```python
from build123d import *

# Parameters (mm, degrees)
CYLINDER004_R     = 1.8
CYLINDER004_DEPTH = 10
CYLINDER005_R     = 1.8
CYLINDER005_DEPTH = 10
CYLINDER002_R     = 1.8
CYLINDER002_DEPTH = 10
CYLINDER003_R     = 1.8
CYLINDER003_DEPTH = 10
CYLINDER001_R     = 2.5
CYLINDER001_DEPTH = 24
CYLINDER_R        = 11
CYLINDER_DEPTH    = 2
BOX_W             = 42.3
BOX_H             = 39.8
BOX_DEPTH         = 42.3


with BuildPart() as cylinder004:
    # Cylinder004 → Cylinder004 (new body)
    with BuildSketch(Plane(origin=(5.65, 0, 36.65), x_dir=(1, 0, 0), z_dir=(0, -1, 0))):
        Circle(CYLINDER004_R)
    extrude(amount=CYLINDER004_DEPTH)


with BuildPart() as cylinder005:
    # Cylinder005 → Cylinder005 (new body)
    with BuildSketch(Plane(origin=(36.65, 0, 36.65), x_dir=(1, 0, 0), z_dir=(0, -1, 0))):
        Circle(CYLINDER005_R)
    extrude(amount=CYLINDER005_DEPTH)


with BuildPart() as cylinder002:
    # Cylinder002 → Cylinder002 (new body)
    with BuildSketch(Plane(origin=(5.65, 0, 5.65), x_dir=(1, 0, 0), z_dir=(0, -1, 0))):
        Circle(CYLINDER002_R)
    extrude(amount=CYLINDER002_DEPTH)


with BuildPart() as cylinder003:
    # Cylinder003 → Cylinder003 (new body)
    with BuildSketch(Plane(origin=(36.65, 0, 5.65), x_dir=(1, 0, 0), z_dir=(0, -1, 0))):
        Circle(CYLINDER003_R)
    extrude(amount=CYLINDER003_DEPTH)


with BuildPart() as cylinder001:
    # Cylinder001 → Cylinder001 (new body)
    with BuildSketch(Plane(origin=(21.15, -2, 21.15), x_dir=(1, 0, 0), z_dir=(0, -1, 0))):
        Circle(CYLINDER001_R)
    extrude(amount=CYLINDER001_DEPTH)


with BuildPart() as cylinder:
    # Cylinder → Cylinder (new body)
    with BuildSketch(Plane(origin=(21.15, 0, 21.15), x_dir=(1, 0, 0), z_dir=(0, -1, 0))):
        Circle(CYLINDER_R)
    extrude(amount=CYLINDER_DEPTH)


with BuildPart() as fusion002:
    # Box → Box (new body)
    with BuildSketch(Plane.XY):
        with Locations((21.15, 19.9)):
            Rectangle(BOX_W, BOX_H)
    extrude(amount=BOX_DEPTH)

    # Fusion: union Cylinder
    add(cylinder.part)

    # Fusion001: union Cylinder001
    add(cylinder001.part)

    # Fusion002: union Cylinder004, Cylinder005, Cylinder002, Cylinder003
    add(cylinder004.part)
    add(cylinder005.part)
    add(cylinder002.part)
    add(cylinder003.part)


solid = fusion002.part
```
Input: part model. Units: mm. Frame: model coordinates. A direction names the side the tool comes from. Give positions to 0.01 mm unless a question says otherwise; leave off trailing zeros. Write each loop counter-clockwise with the first axis right and the second up, starting at its lowest first coordinate (ties: lowest second). Pieces come first, ordered by that corner, then holes. Notation, with made-up numbers: (-30.75, 61) - (-17.75, 61) arc R13 cw to (-17.75, 74) - close; hole circle Ø3 at (88, -18). An arc over 180 degrees is marked (long way). Write item = value, one per line. Start each with the question number.
1. Access query for faces 1 (the flat face through (30, 0, 30)), 2 (the flat face through (0, 20, 21)). Directions: +Z, -Z, +X, -X, +Y, -Y. A direction counts if a zero-diameter tool reaches every point of the face in a straight line with its end or side. Return the directions, or none.
2. First-contact query: pin 1 Ø3 at (x, z) = (36.5, 36.5) entering from -Y; pin 2 Ø1 at (x, z) = (14, 9) entering from -Y; pin 3 Ø3 at (y, z) = (-10.5, 34) entering from +X. Flat tips, straight axial feed; report the tip coordinate or a pass-through.
3. Section query D-D, the plane y = -13. Output: boundary loops of the cut face in (x, z), then the cut area to 3 significant figures.
4. Section query B-B, the plane z = 5.65. Output: boundary loops of the cut face in (x, y).
5. Section query A-A, the plane y = -6. Output: boundary loops of the cut face in (x, z).
6. Ray query, L1, parallel to Y at x = 6, z = 21.5; L2, parallel to Z at x = 7, y = -7; L3, parallel to X at y = -4.5, z = 4. Return the intervals inside material, ascending.
7. Mould query, pull axis X, two halves, no side actions, for faces 3 (the flat face through (6, -10, 37)), 4 (the cylindrical face through (13.04, -0.99, 28.58)), 5 (the cylindrical face through (38.313, -4.93, 35.961)), 6 (the cylindrical face through (38.367, -4.93, 6.191)). Classes: released by +X, released by -X, zero draft, split by the parting line, or undercut.
8. Section query C-C, the plane x = 5.65. Output: boundary loops of the cut face in (y, z), then the cut area to 3 significant figures.
Check sheet entries:
q1.face_1 = -Y
q1.face_2 = +Z, -Z, -X, +Y, -Y
q2.pin_1 = -10
q2.pin_2 = 0
q2.pin_3 = 37.96
q3.outline = circle Ø5 at (21.15, 21.15)
q3.area = 19.6 mm2
q4.outline = (0, 0) - (3.85, 0) - (3.85, -10) - (7.45, -10) - (7.45, 0) - (34.85, 0) - (34.85, -10) - (38.45, -10) - (38.45, 0) - (42.3, 0) - (42.3, 39.8) - (0, 39.8) - close
q5.outline = circle Ø3.6 at (5.65, 5.65); circle Ø3.6 at (5.65, 36.65); circle Ø5 at (21.15, 21.15); circle Ø3.6 at (36.65, 5.65); circle Ø3.6 at (36.65, 36.65)
q6.L1 = 0 to 39.8
q6.L2 = 4.46 to 6.84, 35.46 to 37.84
q6.L3 = 4.93 to 6.37, 35.93 to 37.37
q7.face_3 = zero draft
q7.face_4 = split by the parting line
q7.face_5 = undercut
q7.face_6 = undercut
q8.outline = (-10, 3.85) - (0, 3.85) - (0, 0) - (39.8, 0) - (39.8, 42.3) - (0, 42.3) - (0, 38.45) - (-10, 38.45) - (-10, 34.85) - (0, 34.85) - (0, 7.45) - (-10, 7.45) - close
q8.area = 1,760 mm2
